The listing builds one solid part. Answer for the finished solid, in the listing's coordinates (mm). A direction names the side the tool comes from. Give positions to 0.01 mm unless a question says otherwise; leave off trailing zeros. Loops run counter-clockwise (first coordinate to the right, second up) from the corner with the lowest first, then second, coordinate; pieces in that order, holes last. Notation, with made-up numbers: M 46,43.25 L 89,43.25 A14 ccw 89,58.25 Z; hole C 42.25,-7.75 d10. An arc over 180 degrees is marked long. Use one line per item in the form item = value. Start each with the question number.
1. The part is cut by section B-B (z = -3.5). Write down the section's boundary in (x, y).
2. For faces 1 (the face through (0, 0, 0)), 2 (the face through (-1.097, 24.765, 1.021)), determine the directions among +Z, -Z, +X, -X, +Y, -Y from which every point of the face is accessible in a straight line to the end or side of a thin tool.
3. Each of these flat-tipped pins is pushed along its axis until it touches: pin 1 Ø2 at (x, z) = (3.5, -3) entering from +Y; pin 2 Ø5 at (x, y) = (-3.5, 22) entering from -Z; pin 3 Ø3 at (x, z) = (0.5, -2) entering from -Y; pin 4 Ø5 at (x, y) = (3.5, 22) entering from +Z. Where does it stop, or does it pass through?
4. The part is cut by section C-C (x = 3.25). Write down the section's boundary in (y, z).
5. The part is cut by section D-D (y = 20). Write down the section's boundary in (x, z), and give its area (3 significant figures).
6. The part is cut by section A-A (y = 7.5). Write down the section's boundary in (x, z).
7. The mould has two halves that part along X. Classify faces 3 (the face through (0.46, 24.76, -1.46)), 4 (the face through (-2, 19.3, 1)), 5 (the face through (-2.89, 9.79, -3.77)), 6 (the face through (-0.074, 24.765, -1.746)): released by +X, released by -X, zero draft, split by the parting line, or undercut.
8. Straight lines are drawn through the part: line 1 (Z direction, x = 0.25, y = 18.25); line 2 (Y direction, x = 1, z = -3.25); line 3 (Y direction, x = -1.75, z = 0). For each, find the intervals that lie inside material, in ascending order. Write a range as from..to.
from build123d import *

# Parameters (mm, degrees)
SKETCH1_R           = 6.2
BOSS_EXTRUDE1_DEPTH = 19.5
SKETCH2_R           = 2
BOSS_EXTRUDE2_DEPTH = 2.8
SKETCH3_R           = 0.4
BOSS_EXTRUDE4_DEPTH = 5
CUT_EXTRUDE1_START  = -0.2
SKETCH4_R           = 4.75
SKETCH4_R_2         = 2
CUT_EXTRUDE1_DEPTH  = 0.2
SKETCH5_R           = 0.4
BOSS_EXTRUDE5_DEPTH = 3.5
SKETCH6_R           = 6.2
SKETCH6_R_2         = 4.75
CUT_EXTRUDE2_DEPTH  = 25.614629796
SKETCH7_R           = 9.512731099
CUT_EXTRUDE3_DEPTH  = 29.114320195


with BuildPart() as part:
    # Sketch1 → Boss-Extrude1 (new body)
    with BuildSketch(Plane(origin=(0, 0, 0), x_dir=(1, 0, 0), z_dir=(0, 1, 0))):
        with Locations(Location((0, 0, 0), (0, 0, 270))):
            Circle(SKETCH1_R)
    extrude(amount=BOSS_EXTRUDE1_DEPTH)

    # Sketch2 → Boss-Extrude2 (add)
    with BuildSketch(Plane(origin=(0, 19.5, 0), x_dir=(1, 0, 0), z_dir=(0, 1, 0))):
        with Locations(Location((0, 0, 0), (0, 0, 270))):
            Circle(SKETCH2_R)
    extrude(amount=BOSS_EXTRUDE2_DEPTH)

    # Sketch3 → Boss-Extrude4 (add)
    with BuildSketch(Plane(origin=(0, 22.3, 0), x_dir=(1, 0, 0), z_dir=(0, 1, 0))):
        with Locations(Location((-0.41145274, -0.237271907, 0), (0, 0, 270))):
            Circle(SKETCH3_R)
        with Locations(Location((-0.09128588, 1.346231062, 0), (0, 0, 270))):
            Circle(SKETCH3_R)
        with Locations(Location((0.706061251, 1.146478436, 0), (0, 0, 270))):
            Circle(SKETCH3_R)
        with Locations(Location((1.233716983, 0.516206281, 0), (0, 0, 270))):
            Circle(SKETCH3_R)
        with Locations(Location((1.29013476, -0.30384286, 0), (0, 0, 270))):
            Circle(SKETCH3_R)
        with Locations(Location((0.853764908, -1.000438089, 0), (0, 0, 270))):
            Circle(SKETCH3_R)
        with Locations(Location((0.09128588, -1.307503705, 0), (0, 0, 270))):
            Circle(SKETCH3_R)
        with Locations(Location((-0.706061251, -1.107751078, 0), (0, 0, 270))):
            Circle(SKETCH3_R)
        with Locations(Location((-1.233716983, -0.477478923, 0), (0, 0, 270))):
            Circle(SKETCH3_R)
        with Locations(Location((-1.29013476, 0.342570218, 0), (0, 0, 270))):
            Circle(SKETCH3_R)
        with Locations(Location((-0.853764908, 1.039165447, 0), (0, 0, 270))):
            Circle(SKETCH3_R)
        with Locations(Location((0, 0.516206281, 0), (0, 0, 270))):
            Circle(SKETCH3_R)
        with Locations(Location((0.441742202, -0.237271907, 0), (0, 0, 270))):
            Circle(SKETCH3_R)
    extrude(amount=BOSS_EXTRUDE4_DEPTH)

    # Sketch4 → Cut-Extrude1 (cut)
    with BuildSketch(Plane(origin=(0, 19.5, 0), x_dir=(1, 0, 0), z_dir=(0, 1, 0)).offset(CUT_EXTRUDE1_START)):
        with Locations(Location((0, 0, 0), (0, 0, 270))):
            Circle(SKETCH4_R)
        with Locations(Location((0, 0, 0), (0, 0, 270))):
            Circle(SKETCH4_R_2, mode=Mode.SUBTRACT)
    extrude(amount=CUT_EXTRUDE1_DEPTH, mode=Mode.SUBTRACT)

    # Sketch5 → Boss-Extrude5 (add)
    with BuildSketch(Plane.XZ):
        with Locations(Location((-5.700120356, 0, 0), (0, 0, 90))):
            Circle(SKETCH5_R)
        with Locations(Location((-5.629942415, 0.891695278, 0), (0, 0, 90))):
            Circle(SKETCH5_R)
        with Locations(Location((-4.791405516, 0, 0), (0, 0, 90))):
            Circle(SKETCH5_R)
        with Locations(Location((-4.703373902, 0.914243273, 0), (0, 0, 90))):
            Circle(SKETCH5_R)
        with Locations(Location((-4.703373902, -0.914243273, 0), (0, 0, 90))):
            Circle(SKETCH5_R)
        with Locations(Location((-5.629942415, -0.891695278, 0), (0, 0, 90))):
            Circle(SKETCH5_R)
        with Locations(Location((5.629942415, -0.891695278, 0), (0, 0, 90))):
            Circle(SKETCH5_R)
        with Locations(Location((4.703373902, -0.914243273, 0), (0, 0, 90))):
            Circle(SKETCH5_R)
        with Locations(Location((4.703373902, 0.914243273, 0), (0, 0, 90))):
            Circle(SKETCH5_R)
        with Locations(Location((4.791405516, 0, 0), (0, 0, 90))):
            Circle(SKETCH5_R)
        with Locations(Location((5.629942415, 0.891695278, 0), (0, 0, 90))):
            Circle(SKETCH5_R)
        with Locations(Location((5.700120356, 0, 0), (0, 0, 90))):
            Circle(SKETCH5_R)
    extrude(amount=BOSS_EXTRUDE5_DEPTH)

    # Sketch6 → Cut-Extrude2 (cut, through all)
    with BuildSketch(Plane(origin=(0, 19.5, 0), x_dir=(1, 0, 0), z_dir=(0, 1, 0))):
        Circle(SKETCH6_R)
        with Locations(Location((0, 0, 0), (0, 0, 270))):
            Circle(SKETCH6_R_2, mode=Mode.SUBTRACT)
    extrude(amount=-CUT_EXTRUDE2_DEPTH, mode=Mode.SUBTRACT)

    # Sketch7 → Cut-Extrude3 (cut, through all)
    with BuildSketch(Plane.XZ):
        Circle(SKETCH7_R)
    extrude(amount=CUT_EXTRUDE3_DEPTH, mode=Mode.SUBTRACT)


solid = part.part
Derived:
q1.outline = M -3.21,0 L 3.21,0 L 3.21,19.3 L -3.21,19.3 Z
q2.face_1 = +Z, -Z, +X, -X, -Y
q2.face_2 = +Y
q3.pin_1 = 19.3
q3.pin_2 = -1.73
q3.pin_3 = 0
q3.pin_4 = 1.73
q4.outline = M 0,-3.46 L 19.3,-3.46 L 19.3,3.46 L 0,3.46 Z
q5.outline = C 0,0 d4
q5.area = 12.6 mm2
q6.outline = C 0,0 d9.5
q7.face_3 = undercut
q7.face_4 = zero draft
q7.face_5 = split by the parting line
q7.face_6 = undercut
q8.line_1 = -4.74..4.74
q8.line_2 = 0..19.3
q8.line_3 = 0..22.3
